The listing builds one solid part. Answer for the finished solid, in the listing's coordinates (mm). Give positions to 0.01 mm unless a question says otherwise; leave off trailing zeros. Write each loop counter-clockwise with the first axis right and the second up, starting at its lowest first coordinate (ties: lowest second). Pieces come first, ordered by that corner, then holes.
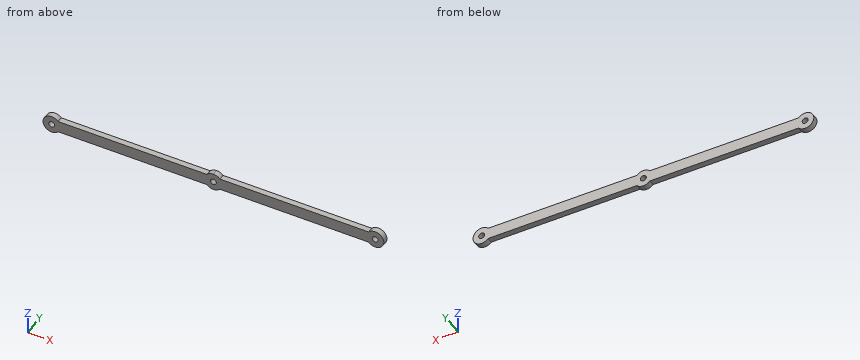
```python
from build123d import *

# Parameters (mm, degrees)
F0_R     = 1.6256
F1_DEPTH = 3.175


with BuildPart() as f1:
    # F0 (on Front) → F1 (new body)
    with BuildSketch(Plane.XZ):
        with BuildLine():
            Line((0, -3.175), (0, 0))
            Line((0, 0), (0, 3.175))
            Line((0, 3.175), (-40.900242, 3.175))
            ThreePointArc((-40.900242, 3.175), (-42.505718, 4.347548), (-44.45, 4.7625))
            Line((-44.45, 4.7625), (-44.45, 1.6256))
            ThreePointArc((-44.45, 1.6256), (-43.300527, 1.149473), (-42.8244, 0))
            ThreePointArc((-42.8244, 0), (-43.300527, -1.149473), (-44.45, -1.6256))
            Line((-44.45, -1.6256), (-44.45, -4.7625))
            ThreePointArc((-44.45, -4.7625), (-42.505718, -4.347548), (-40.900242, -3.175))
            Line((-40.900242, -3.175), (0, -3.175))
        make_face()
        with BuildLine():
            Line((0, 3.175), (0, 0))
            Line((0, 0), (0, -3.175))
            Line((0, -3.175), (40.900242, -3.175))
            ThreePointArc((40.900242, -3.175), (49.2125, 0), (40.900242, 3.175))
            Line((40.900242, 3.175), (0, 3.175))
        make_face()
        with BuildLine():
            ThreePointArc((46.0756, 0), (44.45, -1.6256), (42.8244, 0))
            ThreePointArc((42.8244, 0), (44.45, 1.6256), (46.0756, 0))
        make_face(mode=Mode.SUBTRACT)
        with BuildLine():
            ThreePointArc((-47.999758, -3.175), (-49.2125, 0), (-47.999758, 3.175))
            Line((-47.999758, 3.175), (-88.9, 3.175))
            Line((-88.9, 3.175), (-129.800242, 3.175))
            ThreePointArc((-129.800242, 3.175), (-138.1125, 0), (-129.800242, -3.175))
            Line((-129.800242, -3.175), (-88.9, -3.175))
            Line((-88.9, -3.175), (-47.999758, -3.175))
        make_face()
        with Locations((-133.35, 0)):
            Circle(F0_R, mode=Mode.SUBTRACT)
        with BuildLine():
            Line((-44.45, 1.6256), (-44.45, 4.7625))
            ThreePointArc((-44.45, 4.7625), (-46.394282, 4.347548), (-47.999758, 3.175))
            ThreePointArc((-47.999758, 3.175), (-49.2125, 0), (-47.999758, -3.175))
            ThreePointArc((-47.999758, -3.175), (-46.394282, -4.347548), (-44.45, -4.7625))
            Line((-44.45, -4.7625), (-44.45, -1.6256))
            ThreePointArc((-44.45, -1.6256), (-46.0756, 0), (-44.45, 1.6256))
        make_face()
    extrude(amount=F1_DEPTH)


solid = f1.part
```
Item 1: A cutting plane is placed at C-C, the plane x = -17.5. Give the vertices of the cut face in (y, z) (3 decimals), plus the area to 3 significant figures.
Conclusion:
outline: (-3.175, -3.175) - (0, -3.175) - (0, 3.175) - (-3.175, 3.175) - close
area: 20.2 mm2
Item 2: Each of these flat-tipped pins is pushed along its axis until it touches: P1, Ø4, axis at x = 9, z = 3.5, coming from the +Y side; P2, Ø1, axis at x = -7.5, y = -2, coming from the -Z side (3 decimals); P3, Ø1, axis at x = -89, y = -1.5, coming from the +Z side (3 decimals); P4, Ø1.5, axis at y = -1, z = -3, coming from the -X side. Where does it stop, or does it pass through?
Conclusion:
P1: stops at y = 0
P2: stops at z = -3.175
P3: stops at z = 3.175
P4: stops at x = -137.55
Item 3: A cutting plane is placed at B-B, the plane y = -0.7. Count the separate pieces of the cut face and the enclosed holes in it, plus the area to 3 significant figures.
Conclusion:
separate pieces: 1
enclosed holes: 3
area: 1,210 mm2
Item 4: A cutting plane is placed at A-A, the plane x = -133.35. Give the vertices of the cut face in (y, z) (1 decimal), plus the area to 3 significant figures.
Conclusion:
outline: (-3.2, -4.8) - (0, -4.8) - (0, -1.6) - (-3.2, -1.6) - close; (-3.2, 1.6) - (0, 1.6) - (0, 4.8) - (-3.2, 4.8) - close
area: 19.9 mm2
Item 5: Consider probe 1 along X at (y, z) = (-1.6, -0.25); probe 2 along Z at (x, y) = (-133.35, -1.1); probe 3 along X at (y, z) = (-1.6, -1). Determine where each line is inside the solid, lowest interval first.
Conclusion:
probe 1: x = -138.11 to -134.96, -131.74 to -46.06, -42.84 to 42.84, 46.06 to 49.21
probe 2: z = -4.76 to -1.63, 1.63 to 4.76
probe 3: x = -138.01 to -134.63, -132.07 to -45.73, -43.17 to 43.17, 45.73 to 49.11
